```python
from build123d import *

# Parameters (mm, degrees)
EXTRUDE_1_DEPTH = 3
SKETCH_3_R      = 2.4
EXTRUDE_2_DEPTH = 0.4
EXTRUDE_3_DEPTH = 3.6


with BuildPart() as part:
    # 草图2 → 凸台-拉伸1 (new body)
    with BuildSketch(Plane(origin=(0, 0, 0), x_dir=(1, 0, 0), z_dir=(0, 1, 0))):
        Polygon((0, -2.886751346), (2.5, -1.443375673), (2.5, 1.443375673), (0, 2.886751346), (-2.5, 1.443375673), (-2.5, -1.443375673), align=None)
    extrude(amount=-EXTRUDE_1_DEPTH)

    # 草图3 → 凸台-拉伸2 (add)
    with BuildSketch(Plane.XZ.offset(3)):
        Circle(SKETCH_3_R)
    extrude(amount=EXTRUDE_2_DEPTH)

    # 草图4 → 凸台-拉伸3 (add)
    with BuildSketch(Plane.XZ.offset(3.4)):
        Polygon((0, -3.175426481), (2.75, -1.58771324), (2.75, 1.58771324), (0, 3.175426481), (-2.75, 1.58771324), (-2.75, -1.58771324), align=None)
    extrude(amount=EXTRUDE_3_DEPTH)


solid = part.part
```
Can you work these out from the model? Positions are in its coordinate system, mm. A direction names the side the tool comes from. Give positions to 0.01 mm unless a question says otherwise; leave off trailing zeros. Write each loop counter-clockwise with the first axis right and the second up, starting at its lowest first coordinate (ties: lowest second). Pieces come first, ordered by that corner, then holes. Notation, with made-up numbers: (-5, -37) -> (8, -37) arc R25 ccw to (8, -24) -> close; hole circle Ø3 at (46.25, 69.25). An arc over 180 degrees is marked (long way). Write item = value, one per line.
(1) Suppose I cut it at D-D on z = 0. Write out the boundary of the cut face in (x, y), then the cut area to 3 significant figures.
Worked out:
outline = (-2.75, -7) -> (2.75, -7) -> (2.75, -3.4) -> (2.4, -3.4) -> (2.4, -3) -> (2.5, -3) -> (2.5, 0) -> (-2.5, 0) -> (-2.5, -3) -> (-2.4, -3) -> (-2.4, -3.4) -> (-2.75, -3.4) -> close
area = 36.7 mm^2
(2) Suppose I cut it at C-C on x = -1.55. Write out the boundary of the cut face in (y, z).
Worked out:
outline = (-7, -2.28) -> (-3.4, -2.28) -> (-3.4, -1.83) -> (-3, -1.83) -> (-3, -1.99) -> (0, -1.99) -> (0, 1.99) -> (-3, 1.99) -> (-3, 1.83) -> (-3.4, 1.83) -> (-3.4, 2.28) -> (-7, 2.28) -> close
(3) Suppose I cut it at B-B on y = -5. Write out the boundary of the cut face in (x, z), then the cut area to 3 significant figures.
Worked out:
outline = (-2.75, -1.59) -> (0, -3.18) -> (2.75, -1.59) -> (2.75, 1.59) -> (0, 3.18) -> (-2.75, 1.59) -> close
area = 26.2 mm^2
(4) Suppose I cut it at A-A on z = -2.5. Write out the boundary of the cut face in (x, y), then the cut area to 3 significant figures.
Worked out:
outline = (-1.17, -7) -> (1.17, -7) -> (1.17, -3.4) -> (-1.17, -3.4) -> close; (-0.67, -3) -> (0.67, -3) -> (0.67, 0) -> (-0.67, 0) -> close
area = 12.4 mm^2
(5) I'm going to push flat-ended pins straight in: P1, Ø1.5, axis at x = -0.5, y = -5.5, coming from the -Z side; P2, Ø0.9, axis at y = -1, z = -0.5, coming from the -X side. Where does each tip first touch, or does it pass through?
Worked out:
P1 = -3.18
P2 = -2.5
(6) For faces 1 (the face through (1.29, -3.197, 2.024)), 2 (the face through (2.5, -1, 0)), 3 (the face through (-1.267, -1.479, 2.155)), which set-ups out of +Z, -Z, +X, -X, +Y, -Y let a thin tool reach every point of the face, with its end or its side?
Worked out:
face_1 = none
face_2 = +Z, -Z, +X, +Y
face_3 = +Z, -X, +Y
(7) I need wall thicknesses on probe 1 along Y at (x, z) = (-1.9, -1.75); probe 2 along X at (y, z) = (-1.25, -0.25); probe 3 along Y at (x, z) = (0.5, 2.75). Which ranges of each line are inside material? Lowest first, please. Write a range as from..to.
Worked out:
probe_1 = -7..-3.4, -3..0
probe_2 = -2.5..2.5
probe_3 = -7..-3.4
